Verification items for this drawing (mm, ordinates from the low corner). A direction names the side the tool comes from. Round coordinates to 2 decimals unless told otherwise and drop trailing zeros. Order: outer loops, then holes, each group sorted by start corner. A loop starts at its lowest first (then second) coordinate and runs counter-clockwise, first axis right, second up. Notation, with made-up numbers: M 2,-6 L 26,-6 A23 ccw 26,5 Z; hole C 53,43.25 d9. An arc over 180 degrees is marked long. Return JSON: item names as keys, results as strings. Group by question number.
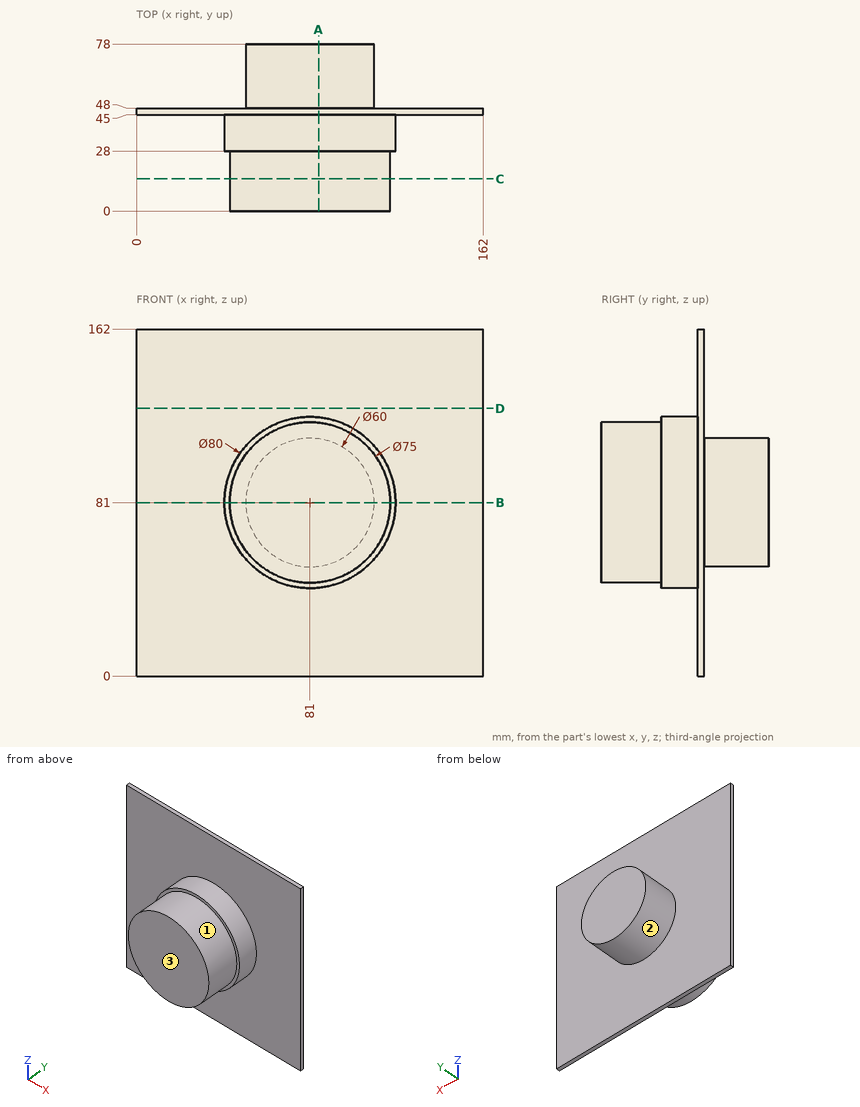
Q1. Section check B-B on z = 81. Record the cut outline in (x, y).
Q2. Depth check by flat-ended pin: pin 1 Ø1 at (y, z) = (54.5, 108) entering from +X; pin 2 Ø8 at (y, z) = (33, 65.5) entering from +X; pin 3 Ø5 at (x, z) = (66.5, 40.5) entering from +Y; pin 4 Ø10 at (x, y) = (122, 57.5) entering from -Z. Enter the tip coordinate at first touch or a pass-through.
Q3. Set-up check for the marked faces 1, 2 and 3: record each of +Z, -Z, +X, -X, +Y, -Y from which the full face is reachable in a straight line by a thin tool's end or side.
Q4. Section check A-A on x = 85. Record the cut outline in (y, z).
Q5. Section check D-D on z = 125. Record the cut outline in (x, y).
Q6. Section check C-C on y = 15. Record the cut outline in (x, z), plus the area to 3 significant figures.
Q7. Material ranges on line 1 along Y through (x, z) = (38, 20); line 2 along Z through (x, y) = (82, 34.5); line 3 along Z through (x, y) = (91.5, 59), recorded low to high.
Geometry check:
{
 "1": {"outline": "M 0,45 L 41,45 L 41,28 L 43.5,28 L 43.5,0 L 118.5,0 L 118.5,28 L 121,28 L 121,45 L 162,45 L 162,48 L 111,48 L 111,78 L 51,78 L 51,48 L 0,48 Z"},
 "2": {"pin 1": "stops at x = 95.06", "pin 2": "stops at x = 119.31", "pin 3": "stops at y = 48", "pin 4": "passes through"},
 "3": {"face 1": "-Y", "face 2": "+Y", "face 3": "+Z, -Z, +X, -X, -Y"},
 "4": {"outline": "M 0,43.71 L 28,43.71 L 28,41.2 L 45,41.2 L 45,0 L 48,0 L 48,51.27 L 78,51.27 L 78,110.73 L 48,110.73 L 48,162 L 45,162 L 45,120.8 L 28,120.8 L 28,118.29 L 0,118.29 Z"},
 "5": {"outline": "M 0,45 L 162,45 L 162,48 L 0,48 Z"},
 "6": {"outline": "C 81,81 d75", "area": "4,420 mm^2"},
 "7": {"line 1": "y = 45 to 48", "line 2": "z = 41.01 to 120.99", "line 3": "z = 52.9 to 109.1"}
}
